Source: CAD feature listing. Evaluate the final solid. Frame: model axes, mm. A direction names the side the tool comes from. Round coordinates to 2 decimals unless told otherwise and drop trailing zeros. Loops run counter-clockwise (first coordinate to the right, second up) from the corner with the lowest first, then second, coordinate; pieces in that order, holes last. Notation, with made-up numbers: (86, 57) - (98, 57) arc R22 ccw to (98, 82) - close; hole circle Ø8 at (60, 73). An arc over 180 degrees is marked (long way). Write item = value, one per line. Start each with the question number.
Autodesk Inventor part; units mm, degrees
ref_plane "YZ Plane" through (0, 0, 0) normal (1, 0, 0) x (0, 1, 0)
ref_plane "XZ Plane" through (0, 0, 0) normal (0, 1, 0) x (-1, 0, 0)
ref_plane "XY Plane" through (0, 0, 0) normal (0, 0, 1) x (1, 0, 0)
sketch "スケッチ1" plane through (0, 0, 0) normal (0, 0, 1) x (1, 0, 0)
  circle A0 centre (0, 0) radius 10.5 construction
  line L0 (-12, 10.583) -> (-12, -10.583) construction
  arc A1 (0, 16) -> (-12, 10.583) centre (0, 0) ccw construction
  line L1 (0, 16) -> (33.5167, 16) construction
  line L2 (33.5167, 16) -> (33.5167, -16) construction
  line L3 (33.5167, -16) -> (0, -16) construction
  arc A2 (-12, -10.583) -> (0, -16) centre (0, 0) ccw construction
  circle A3 centre (0, 8.5) radius 1.35
  circle A4 centre (-8.5, 0) radius 1.35
  circle A5 centre (0, -8.5) radius 1.35
  circle A6 centre (8.5, 0) radius 1.35
  circle A7 centre (0, 0) radius 5.05
  circle A8 centre (0, 0) radius 16 construction
  line L4 (-21.5, 6) -> (-19, 6) construction
  line L5 (-19, 6) -> (-19, -6) construction
  line L6 (-19, -6) -> (-21.5, -6) construction
  line L7 (-21.5, -6) -> (-21.5, 6) construction
  circle A9 centre (0, 0) radius 19 construction
  line L8 (-18.95, 6.05) -> (-21.55, 6.05) construction
  line L9 (-21.55, 6.05) -> (-21.55, -6.05) construction
  line L10 (-21.55, -6.05) -> (-18.95, -6.05) construction
  line L11 (-18.95, -6.05) -> (-18.95, 6.05) construction
  circle A10 centre (-21.55, 5) radius 1.05 construction
  line L12 (-18.95, 6.05) -> (-21.55, 6.05)
  arc A11 (-21.55, 6.05) -> (-21.55, 3.95) centre (-21.55, 5) ccw
  line L13 (-21.55, 3.95) -> (-21.55, -3.95)
  line L14 (-20.25, 6.05) -> (-20.25, -6.05) construction
  line L15 (-21.55, 0) -> (-19, 0) construction
  arc A12 (-21.55, -3.95) -> (-21.55, -6.05) centre (-21.55, -5) ccw
  line L16 (-21.55, -6.05) -> (-18.95, -6.05)
  line L17 (-18.95, 3.95) -> (-18.95, -3.95)
  arc A13 (-18.95, 3.95) -> (-18.95, 6.05) centre (-18.95, 5) ccw
  arc A14 (-18.95, -6.05) -> (-18.95, -3.95) centre (-18.95, -5) ccw
  line L18 (-24, 6) -> (-24, -6)
  circle A15 centre (-21.5, 13) radius 1.55
  circle A16 centre (-21.5, -13) radius 1.55
  line L19 (-24, 16) -> (-21.201, 16)
  line L20 (-24, -16) -> (-21.201, -16)
  arc A17 (2.2701, -11.2737) -> (2.2701, 11.2737) centre (0, 0) ccw
  line L21 (-24, 16) -> (-24, 6)
  circle A18 centre (-21.5, 13) radius 3 construction
  line L22 (-24, -16) -> (-24, -6)
  line L23 (-21.201, 16) -> (2.2701, 11.2737)
  line L24 (2.2701, -11.2737) -> (-21.201, -16)
  point P0 (-12, 0)
  point P1 (-20.275, 0)
  dimension "d29" = 2.1
  dimension "d0" = 21
  dimension "d1" = 16
  dimension "d2" = 12
  dimension "d3" = 8.5
  dimension "d4" = 2.7
  dimension "d7" = 360
  dimension "d9" = 10.1
  dimension "d10" = 2.5
  dimension "d11" = 3
  dimension "d27" = 10
  dimension "d30" = 0.05
  dimension "d31" = 7
  dimension "d33" = 3.1
  dimension "d41" = 2.5
  dimension "d43" = 1
extrude "押し出し1" add sketch "スケッチ1" along normal blind 1.5
equation "\"d27\" = d21"
equation "\"d31\" = d23"
properties part number "肩_サブフレーム_1_1" material "アルミニウム 2014-T4"
(1) Cut plane D-D (y = 4.5). Output: boundary loops of the cut face in (x, z).
(2) Cut plane B-B (y = 13). Output: boundary loops of the cut face in (x, z), and give its area (3 significant figures).
(3) Cut plane A-A (z = 0.9). State how many separate pieces and enclosed holes the cut face has, and give its area (3 significant figures).
(4) Access query for faces 4 (the face through (-10, 0, 1.5)), 5 (the face through (-20, 6.05, 1)). Directions: +Z, -Z, +X, -X, +Y, -Y. A direction counts if a zero-diameter tool reaches every point of the face in a straight line with its end or side. Return the directions, or none.
(5) Mould query, pull axis Y, two halves, no side actions, for faces 1 (the face through (-9.63, 13.67, 0.74)), 2 (the face through (-10, 0, 0)), 3 (the face through (-17.9, -5, 0.7)). Classes: +Y half, -Y half, draft (parallel to the pull), parting line (faces both ways), or undercut.
(6) Cut plane C-C (x = 0). Output: boundary loops of the cut face in (y, z), and give its area (3 significant figures).
(7) Material intervals for line 1 along Y through (x, z) = (-21.5, 0.4); line 2 along Y through (x, z) = (0, 0.45); line 3 along Y through (x, z) = (-3, 1.4), sorted ascending. Write a range as from..to.
Solution:
q1.outline = (-24, 0) - (-22.47, 0) - (-22.47, 1.5) - (-24, 1.5) - close; (-18.03, 0) - (-2.29, 0) - (-2.29, 1.5) - (-18.03, 1.5) - close; (2.29, 0) - (10.58, 0) - (10.58, 1.5) - (2.29, 1.5) - close
q2.outline = (-24, 0) - (-23.05, 0) - (-23.05, 1.5) - (-24, 1.5) - close; (-19.95, 0) - (-6.3, 0) - (-6.3, 1.5) - (-19.95, 1.5) - close
q2.area = 21.9 mm^2
q3.separate_pieces = 1
q3.enclosed_holes = 8
q3.area = 729 mm^2
q4.face_4 = +Z, +X, -X, +Y, -Y
q4.face_5 = +Z, -Z
q5.face_1 = +Y half
q5.face_2 = draft
q5.face_3 = undercut
q6.outline = (-11.73, 0) - (-9.85, 0) - (-9.85, 1.5) - (-11.73, 1.5) - close; (-7.15, 0) - (-5.05, 0) - (-5.05, 1.5) - (-7.15, 1.5) - close; (5.05, 0) - (7.15, 0) - (7.15, 1.5) - (5.05, 1.5) - close; (9.85, 0) - (11.73, 0) - (11.73, 1.5) - (9.85, 1.5) - close
q6.area = 11.9 mm^2
q7.line_1 = -16..-14.55, -11.45..-6.05, 6.05..11.45, 14.55..16
q7.line_2 = -11.73..-9.85, -7.15..-5.05, 5.05..7.15, 9.85..11.73
q7.line_3 = -12.33..-4.06, 4.06..12.33
